The listing builds one solid part. Answer for the finished solid, in the listing's coordinates (mm). A direction names the side the tool comes from. Round coordinates to 2 decimals unless told otherwise and drop trailing zeros. Order: outer loops, then holes, each group sorted by start corner. A loop starts at its lowest first (then second) coordinate and runs counter-clockwise, first axis right, second up. Notation, with made-up numbers: (-10, 23.5) -> (49, 23.5) arc R34 cw to (49, 57.5) -> close; hole circle Ø9 at (69.25, 3). An arc over 180 degrees is marked (long way). Return JSON: item names as keys, results as strings. Group by question number.
(1) Consider line 1 (Z direction, x = -24.5, y = 29); line 2 (Y direction, x = -35, z = 9); line 3 (X direction, y = 67.5, z = 8). Determine where each line is inside the solid, lowest interval first. Write a range as [from, to].
(2) The part is cut by section C-C (x = 6.5). Determine the outline of the cut face in (y, z), plus the area to 4 significant figures.
(3) The part is cut by section D-D (z = 2). Determine the outline of the cut face in (x, y), plus the area to 3 significant figures.
(4) Which of the six approach directions +Z, -Z, +X, -X, +Y, -Y give full straight-line access (tool end or side, diameter ignored) to faces 1 (the face through (-35, -63, 15.259)), 2 (the face through (22.208, -63, -42)), 3 (the face through (2, 16, -38.638)), 4 (the face through (-22, -49.9, -39)), 5 (the face through (31, -74.9, -42))?
(5) Each of these flat-tipped pins is pushed along its axis until it touches: pin 1 (10 mm diameter, centred on x = -30.5, z = -29, fed in from -Y); pin 2 (3 mm diameter, centred on x = -36, y = -62.5, fed in from -Z); pin 3 (10 mm diameter, centred on y = 46.5, z = -26, fed in from +X). Where does it stop, or does it pass through?
(6) The part is cut by section B-B (y = 30). Determine the outline of the cut face in (x, z), plus the area to 3 significant figures.
(7) The part is cut by section A-A (y = -61.5). Determine the outline of the cut face in (x, z), plus the area to 3 significant figures.
from build123d import *

# Parameters (mm, degrees)
F0_W     = 16.86
F0_H     = 6.1000012737
F1_DEPTH = 74.9
F2_DEPTH = 75.1
F3_R     = 3
F5_DEPTH = 25


with BuildPart() as f1:
    # F0 (on Front) → F1 (new body)
    with BuildSketch(Plane.XZ):
        Polygon((-32.5276732162, 32.1178423136), (-38.6276732162, 32.1178423136), (-38.444462499, 15.2623822779), (-32.5276732162, 15.3266949223), align=None)
        Polygon((-32.5276732162, 15.3266949223), (-38.444462499, 15.2623822779), (-37.7922914511, -44.7376177221), (22.2077085489, -44.7376177221), (22.2077085489, -38.6376164485), (-32.5276732162, -38.6376164485), align=None)
        with Locations((30.6377085489, -41.6876170853)):
            Rectangle(F0_W, F0_H)
    extrude(amount=F1_DEPTH)

    # F2 (add): a face of the model
    f2_faces = [f1.faces().sort_by_distance(p)[0] for p in [
        (-35.5776732162, 0, 31.0249866925),
    ]]
    extrude(f2_faces, amount=F2_DEPTH)

    # F3
    f3_edges = [f1.edges().sort_by_distance(p)[0] for p in [
        (-32.527673, 0.1, 32.117842),
        (-38.627673, 0.1, 32.117842),
        (39.067709, 0.1, -44.737618),
        (39.067709, 0.1, -38.637616),
    ]]
    fillet(f3_edges, radius=F3_R)

    # F4 (on face) → F5 (cut)
    with BuildSketch(Plane.XZ.offset(74.9)):
        Polygon((-32.5276732162, 15.2588381996), (-38.4444239765, 15.2588381996), (-37.7922914511, -44.7376177221), (22.2077085489, -44.7376177221), (22.2077085489, -38.6376164485), (-32.5276732162, -38.6376164485), (-32.5276732162, -35.7810780406), align=None)
    extrude(amount=-F5_DEPTH, mode=Mode.SUBTRACT)


solid = f1.part
Answer below:
{
 "1": {"line 1": "z = [-44.74, -38.64]", "line 2": "y = [-49.9, 75.1]", "line 3": "x = [-38.37, -32.53]"},
 "2": {"outline": "(-49.9, -44.74) -> (75.1, -44.74) -> (75.1, -38.64) -> (-49.9, -38.64) -> close", "area": "762.5 mm²"},
 "3": {"outline": "(-38.3, -49.9) -> (-32.53, -49.9) -> (-32.53, 75.1) -> (-38.3, 75.1) -> close", "area": "722 mm²"},
 "4": {"face 1": "-Z, +X, -X, -Y", "face 2": "+Z, -Z, -X, -Y", "face 3": "+Z, +X, +Y, -Y", "face 4": "-Z, -X, -Y", "face 5": "+Z, -Z, +X, -X, -Y"},
 "5": {"pin 1": "stops at y = -49.9", "pin 2": "stops at z = 15.26", "pin 3": "stops at x = -32.53"},
 "6": {"outline": "(-38.59, 29.09) -> (-37.79, -44.74) -> (36.07, -44.74) arc R3 ccw to (39.07, -41.74) -> (39.07, -41.64) arc R3 ccw to (36.07, -38.64) -> (-32.53, -38.64) -> (-32.53, 29.12) arc R3 ccw to (-35.53, 32.12) -> (-35.59, 32.12) arc R3 ccw to start", "area": "866 mm²"},
 "7": {"outline": "(-38.59, 29.09) -> (-38.44, 15.26) -> (-32.53, 15.26) -> (-32.53, 29.12) arc R3 ccw to (-35.53, 32.12) -> (-35.59, 32.12) arc R3 ccw to start; (22.21, -44.74) -> (36.07, -44.74) arc R3 ccw to (39.07, -41.74) -> (39.07, -41.64) arc R3 ccw to (36.07, -38.64) -> (22.21, -38.64) -> close", "area": "196 mm²"}
}
